Could you check a few things on this model? Use its own coordinates, in mm. Face numbers are marked on the shaded views. A direction names the side the tool comes from. Round coordinates to 2 decimals unless told otherwise and drop trailing zeros. Loops run counter-clockwise (first coordinate to the right, second up) from the corner with the lowest first, then second, coordinate; pieces in that order, holes last. Notation, with made-up numbers: (38.25, 66) -> (71.25, 66) arc R17 cw to (71.25, 75) -> close; hole circle Ø5 at (60, 89). An arc over 180 degrees is marked (long way). One line per item, written item: value.
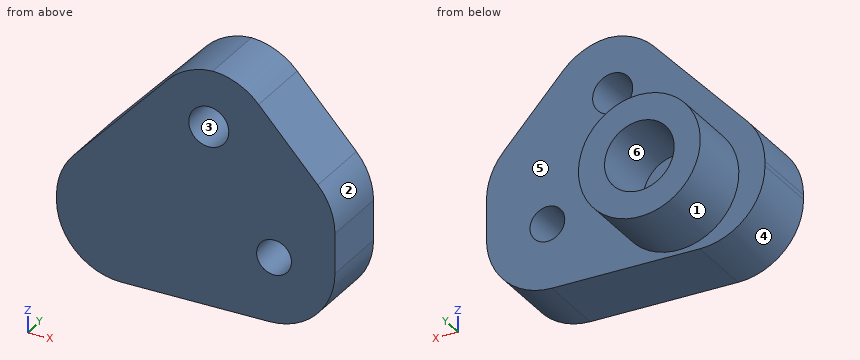
from build123d import *

# Parameters (mm, degrees)
BOSS_EXTRU_1_DEPTH      = 8
CONG_1_R                = 7.5
ENL_V_MAT_EXTRU_1_REACH = 32.467
ESQUISSE2_R             = 2
ESQUISSE2_R_2           = 2.3
ESQUISSE3_R             = 7
ESQUISSE3_R_2           = 4
BOSS_EXTRU_2_DEPTH      = 8
CONG_2_R                = 7.5


with BuildPart() as part:
    # Esquisse1 → Boss.-Extru.1 (new body)
    with BuildSketch(Plane(origin=(0, 0, 0), x_dir=(1, 0, 0), z_dir=(0, 1, 0))):
        Polygon((-10, -3.5), (5, -19.5), (11, -19.5), (22, -7.5), (22, 7.5), (-10, 7.5), align=None)
    extrude(amount=BOSS_EXTRU_1_DEPTH)

    # Congé1
    cong_1_edges = [part.edges().sort_by_distance(p)[0] for p in [
        (-10, 4, -7.5),
        (22, 4, -7.5),
    ]]
    fillet(cong_1_edges, radius=CONG_1_R)

    # Esquisse2 → Enlèv. mat.-Extru.1 (cut, up to next)
    with BuildSketch(Plane(origin=(0, 8, 0), x_dir=(1, 0, 0), z_dir=(0, 1, 0)), mode=Mode.PRIVATE) as enl_v_mat_extru_1_sk1:
        with Locations(Location((15, 0, 0), (0, 0, 270))):
            Circle(ESQUISSE2_R)
    enl_v_mat_extru_1_tool1 = extrude(enl_v_mat_extru_1_sk1.sketch, amount=-ENL_V_MAT_EXTRU_1_REACH, mode=Mode.PRIVATE) & part.part
    # Esquisse2 → Enlèv. mat.-Extru.1 (cut, up to next)
    with BuildSketch(Plane(origin=(0, 8, 0), x_dir=(1, 0, 0), z_dir=(0, 1, 0)), mode=Mode.PRIVATE) as enl_v_mat_extru_1_sk2:
        with Locations(Location((7.5, -12.990381057, 0), (0, 0, 270))):
            Circle(ESQUISSE2_R_2)
    enl_v_mat_extru_1_tool2 = extrude(enl_v_mat_extru_1_sk2.sketch, amount=-ENL_V_MAT_EXTRU_1_REACH, mode=Mode.PRIVATE) & part.part
    add(enl_v_mat_extru_1_tool1.solids().sort_by_distance((15, 8, 0))[0], mode=Mode.SUBTRACT)
    add(enl_v_mat_extru_1_tool2.solids().sort_by_distance((7.5, 8, 12.990381))[0], mode=Mode.SUBTRACT)

    # Esquisse3 → Boss.-Extru.2 (add)
    with BuildSketch(Plane(origin=(0, 8, 0), x_dir=(1, 0, 0), z_dir=(0, 1, 0))):
        with Locations(Location((0, 0, 0), (0, 0, 270))):
            Circle(ESQUISSE3_R)
        with Locations(Location((0, 0, 0), (0, 0, 270))):
            Circle(ESQUISSE3_R_2, mode=Mode.SUBTRACT)
    extrude(amount=BOSS_EXTRU_2_DEPTH)

    # Congé2
    # the kernel refuses this fillet: 7.5 mm, written as the material it takes off along each edge
    with BuildSketch(Plane(origin=(22, -7.293444198, 7.5), x_dir=(-0.6757246285173467, 0, 0.7371541402007411), z_dir=(0, 1, 0))) as cong_2_piece_1:
        with BuildLine():
            CenterArc((CONG_2_R * 0.388983690555, -CONG_2_R), CONG_2_R, 90, 42.510447078)
            Line((-CONG_2_R * 0.286740937963, -CONG_2_R * 0.262845859799), (0, 0))
            Line((0, 0), (CONG_2_R * 0.388983690555, 0))
        make_face()
    extrude(amount=22.586888396, mode=Mode.SUBTRACT)
    with BuildSketch(Plane(origin=(11, -8.248157181, 19.5), x_dir=(-1, 0, 0), z_dir=(0, 1, 0))) as cong_2_piece_2:
        with BuildLine():
            CenterArc((CONG_2_R * 0.439901716342, -CONG_2_R), CONG_2_R, 90, 47.489552922)
            Line((-CONG_2_R * 0.297252423859, -CONG_2_R * 0.324275371483), (0, 0))
            Line((0, 0), (CONG_2_R * 0.439901716342, 0))
        make_face()
    extrude(amount=24.496314363, mode=Mode.SUBTRACT)
    with BuildSketch(Plane(origin=(5, -8.123100234, 19.5), x_dir=(-0.6839411288813303, 0, -0.7295372041400847), z_dir=(0, 1, 0))) as cong_2_piece_3:
        with BuildLine():
            CenterArc((CONG_2_R * 0.433232012466, -CONG_2_R), CONG_2_R, 90, 46.847610266)
            Line((-CONG_2_R * 0.296305191674, -CONG_2_R * 0.316058871119), (0, 0))
            Line((0, 0), (CONG_2_R * 0.433232012466, 0))
        make_face()
    extrude(amount=24.246200467, mode=Mode.SUBTRACT)
    with BuildSketch(Plane(origin=(-10, -7.414640249, 3.5), x_dir=(0, 0, -1), z_dir=(0, 1, 0))) as cong_2_piece_4:
        with BuildLine():
            CenterArc((CONG_2_R * 0.395447479964, -CONG_2_R), CONG_2_R, 90, 43.152389734)
            Line((-CONG_2_R * 0.288493648917, -CONG_2_R * 0.27046279586), (0, 0))
            Line((0, 0), (CONG_2_R * 0.395447479964, 0))
        make_face()
    extrude(amount=22.829280499, mode=Mode.SUBTRACT)


solid = part.part
(1) If we section it at D-D, the plane y = 10.5: Please give me the cut outline in (x, z).
Recorded:
outline: circle Ø14 at (0, 0); hole circle Ø8 at (0, 0)
(2) Thinking about a two-plate mould opening in Z: for the marked faces 3, 4, 5 and 6, which applies, released by +Z, released by -Z, zero draft, split by the parting line, or undercut?
Recorded:
face 3: undercut
face 4: released by -Z
face 5: zero draft
face 6: undercut
(3) I'm going to push flat-ended pins straight in: pin 1 Ø2.5 at (x, z) = (15, 0) entering from +Y; pin 2 Ø6 at (x, z) = (-4, 12) entering from +Y; pin 3 Ø13.5 at (x, z) = (-1, 8) entering from +Y. Where does each tip first touch, or does it pass through?
Recorded:
pin 1: through
pin 2: y = 8
pin 3: y = 16
(4) If I drill on L1, parallel to X at y = 5.5, z = 0; L2, parallel to X at y = 10, z = 0; L3, parallel to Y at x = -2.5, z = 8.5, over which ranges is the centre line in solid material (lowest first)?
Recorded:
L1: -10 to 13, 17 to 22
L2: -7 to -4, 4 to 7
L3: 0 to 8
(5) For the marked faces 1 and 2, which set-ups out of +Z, -Z, +X, -X, +Y, -Y let a thin tool reach every point of the face, with its end or its side?
Recorded:
face 1: +Y
face 2: +Z, +X, +Y, -Y
(6) If we section it at C-C, the plane y = 2.5: Please give me the cut outline in (x, z).
Recorded:
outline: (-10, 0) arc R7.5 ccw to (-2.5, -7.5) -> (14.5, -7.5) arc R7.5 ccw to (22, 0) -> (22, 4.58) arc R7.5 ccw to (20.03, 9.65) -> (13.23, 17.07) arc R7.5 ccw to (7.97, 19.49) arc R7.5 ccw to (2.78, 17.13) -> (-7.97, 5.66) arc R7.5 ccw to (-10, 0.53) -> close; hole circle Ø4.6 at (7.5, 12.99); hole circle Ø4 at (15, 0)
(7) If we section it at B-B, the plane z = 1.5: Please give me the cut outline in (x, y).
Recorded:
outline: (-9.94, 0) -> (13.68, 0) -> (13.68, 8) -> (6.84, 8) -> (6.84, 16) -> (3.71, 16) -> (3.71, 8) -> (-3.71, 8) -> (-3.71, 16) -> (-6.84, 16) -> (-6.84, 8) -> (-9.94, 8) -> close; (16.32, 0) -> (22, 0) -> (22, 8) -> (16.32, 8) -> close
(8) If we section it at A-A, the plane x = 7.5: Please give me the cut outline in (y, z), then the cut area to 3 significant figures.
Recorded:
outline: (0, -7.5) -> (8, -7.5) -> (8, 10.69) -> (0, 10.69) -> close; (0, 15.29) -> (8, 15.29) -> (8, 19.46) -> (0, 19.46) -> close
area: 179 mm²
